Geometry check sheet. Reference: the model listing, model coordinates, mm. A direction names the side the tool comes from. Give positions to 0.01 mm unless a question says otherwise; leave off trailing zeros. Write each loop counter-clockwise with the first axis right and the second up, starting at its lowest first coordinate (ties: lowest second). Pieces come first, ordered by that corner, then holes.
(1) Cross-section at D-D (x = 34). Record the boundary of the cut face in (y, z).
(2) Depth check by flat-ended pin: P1, Ø4, axis at x = 21.5, z = 17, coming from the -Y side; P2, Ø6, axis at x = -26.5, y = 59.5, coming from the -Z side; P3, Ø14.5, axis at x = 20.2, z = 34.88, coming from the -Y side; P4, Ø5.5, axis at x = 20.2, z = -36.77, coming from the +Y side. Enter the tip coordinate at first touch or a pass-through.
(3) Cross-section at A-A (x = 0). Record the boundary of the cut face in (y, z), and give its area (3 significant figures).
(4) Tool access check on faces 4 (the cylindrical face through (0.13, 74.96, 17.68)), 5 (the flat face through (-40, 0, 0)), 6 (the flat face through (-7, 46.828, 6)), 7 (the flat face through (1, 73.811, 34)), 8 (the flat face through (1, 53, -23.514)). Record the directions out of +Z, -Z, +X, -X, +Y, -Y that give a thin tool (end or side, any length) a straight path to the whole face; none if there is none.
(5) Mould release check, pull along X, two halves, no side actions. Record for faces 1 (the flat face through (-1, 89, -44.322)), 2 (the cylindrical face through (45.34, 51.22, -10.48)), 3 (the flat face through (-30.458, 23, 0)): +X half, -X half, draft (parallel to the pull), parting line (faces both ways), or undercut.
(6) Cross-section at C-C (y = 8). Record the boundary of the cut face in (x, z), and give its area (3 significant figures).
(7) Thickness scan on line 1 along X through (y, z) = (14, -15.5); line 2 along X through (y, z) = (14, 6); line 3 along X through (y, z) = (28.5, -10.5). Record the ranges inside material, lowest first.
(8) Cross-section at B-B (z = 0). Record the boundary of the cut face in (x, y), and give its area (3 significant figures).
```python
from build123d import *

# Parameters (mm, degrees)
F0_W     = 99.5807871222
F0_H     = 88.644169271
F1_DEPTH = 103.886
F2_W     = 73.8110467792
F2_H     = 20.8082981408
F3_DEPTH = 202.184
F4_R     = 4.5190102714
F5_DEPTH = 183.388
F6_W     = 62.2652955353
F6_H     = 46.8279197812
F7_DEPTH = 52.07
F9_DEPTH = 124.46


with BuildPart() as f1:
    # F0 (on Front) → F1 (new body)
    with BuildSketch(Plane.XZ):
        Rectangle(F0_W, F0_H)
    extrude(amount=-F1_DEPTH)

    # F2 (on face) → F3 (cut)
    with BuildSketch(Plane.YZ.offset(49.7903935611)):
        with Locations((36.9055233896, 33.9179355651)):
            Rectangle(F2_W, F2_H)
        with Locations((36.9055233896, -33.9179355651)):
            Rectangle(F2_W, F2_H)
    extrude(amount=-F3_DEPTH, mode=Mode.SUBTRACT)

    # F4 (on Front) → F5 (cut)
    with BuildSketch(Plane.XZ):
        with Locations((-17.0435514301, 34.876152873)):
            Circle(F4_R)
        with Locations((20.1997645199, 34.876152873)):
            Circle(F4_R)
        with Locations((-17.0435514301, -36.7698818445)):
            Circle(F4_R)
        with Locations((20.1997645199, -36.7698818445)):
            Circle(F4_R)
        with Locations((-39.168164134, 14.0042221174)):
            Circle(F4_R)
        with Locations((-39.168164134, -12.4670416117)):
            Circle(F4_R)
        with Locations((41.0307683051, 14.0451472253)):
            Circle(F4_R)
        with Locations((41.0307683051, -11.8357995525)):
            Circle(F4_R)
    extrude(amount=-F5_DEPTH, mode=Mode.SUBTRACT)

    # F6 (on face) → F7 (cut)
    with BuildSketch(Plane.XY.offset(23.5137864947)):
        with Locations((0.6743837148, 23.4139598906)):
            Rectangle(F6_W, F6_H)
    extrude(amount=-F7_DEPTH, mode=Mode.SUBTRACT)

    # F8 (on face) → F9 (cut)
    with BuildSketch(Plane.XZ.offset(-46.8279197812)):
        with BuildLine():
            Line((-4.445, 4.3847536734), (-14.7820186248, 4.3847536734))
            ThreePointArc((-14.7820186248, 4.3847536734), (-18.4844560039, -0.342391801), (-14.0998682729, -4.4447493319))
            Line((-14.0998682729, -4.4447493319), (-14.0055365282, -4.4447501768))
            Line((-14.0055365282, -4.4447501768), (-4.445, -4.444835806))
            Line((-4.445, -4.444835806), (-4.445, -14.7025363844))
            ThreePointArc((-4.445, -14.7025363844), (3.51265e-05, -19.1475363843), (4.4449999994, -14.7024661314))
            Line((4.4449999994, -14.7024661314), (4.4448378792, -4.4449154281))
            Line((4.4448378792, -4.4449154281), (13.8872975972, -4.4449999998))
            ThreePointArc((13.8872975972, -4.4449999998), (18.3172518615, 0.3659001816), (13.1579813752, 4.3847536734))
            Line((13.1579813752, 4.3847536734), (4.4446983265, 4.3847536734))
            Line((4.4446983265, 4.3847536734), (4.4445593988, 13.1748796689))
            ThreePointArc((4.4445593988, 13.1748796689), (0.0312927488, 17.6823534639), (-4.445, 13.2374636156))
            Line((-4.445, 13.2374636156), (-4.445, 4.3847536734))
        make_face()
    extrude(amount=-F9_DEPTH, mode=Mode.SUBTRACT)


solid = f1.part
```
Reply:
1. outline: (0, -23.51) - (73.81, -23.51) - (73.81, -44.32) - (103.89, -44.32) - (103.89, 44.32) - (73.81, 44.32) - (73.81, 23.51) - (0, 23.51) - close
2. P1: stops at y = 46.83
2. P2: stops at z = -23.51
2. P3: stops at y = 73.81
2. P4: passes through
3. outline: (46.83, -23.51) - (73.81, -23.51) - (73.81, -44.32) - (103.89, -44.32) - (103.89, -19.15) - (46.83, -19.15) - close; (46.83, 17.68) - (103.89, 17.68) - (103.89, 44.32) - (73.81, 44.32) - (73.81, 23.51) - (46.83, 23.51) - close
3. area: 1,830 mm2
4. face 4: +Y, -Y
4. face 5: +Z, -Z, +X, -X, -Y
4. face 6: +Z, -Z, -Y
4. face 7: +Z, +X, -X, -Y
4. face 8: -Z, +X, -X, -Y
5. face 1: draft
5. face 2: undercut
5. face 3: undercut
6. outline: (-49.79, -23.51) - (-30.46, -23.51) - (-30.46, 23.51) - (-49.79, 23.51) - close; (31.81, -23.51) - (49.79, -23.51) - (49.79, 23.51) - (31.81, 23.51) - close; hole circle Ø9.04 at (-39.17, -12.47); hole circle Ø9.04 at (-39.17, 14); hole circle Ø9.04 at (41.03, -11.84); hole circle Ø9.04 at (41.03, 14.05)
6. area: 1,500 mm2
7. line 1: x = -49.79 to -42.52, -35.82 to -30.46, 31.81 to 38.39, 43.68 to 49.79
7. line 2: x = -49.79 to -30.46, 31.81 to 49.79
7. line 3: x = -49.79 to -43.24, -35.1 to -30.46, 31.81 to 36.71, 45.35 to 49.79
8. outline: (-49.79, 0) - (-30.46, 0) - (-30.46, 46.83) - (-18.5, 46.83) - (-18.5, 103.89) - (-49.79, 103.89) - close; (18.33, 46.83) - (31.81, 46.83) - (31.81, 0) - (49.79, 0) - (49.79, 103.89) - (18.33, 103.89) - close
8. area: 5,330 mm2
